The model under review builds one solid part; all positions refer to its coordinate system, in mm. Coordinates: 2 decimals unless noted, no trailing zeros. Loops run counter-clockwise (first coordinate to the right, second up) from the corner with the lowest first, then second, coordinate; pieces in that order, holes last. Notation, with made-up numbers: M -22,-11.75 L 11,-11.75 A33 ccw 11,23.25 Z; hole C -18.5,-37.75 d4. An arc over 180 degrees is marked long. Use one line per item in the form item = value.
```python
from build123d import *

# Parameters (mm, degrees)
F1_W      = 22
F1_H      = 9
F2_DEPTH  = 25
F2_FACE_W = 22
F2_FACE_H = 9
F3_DEPTH  = 100
F4_R      = 5
F5_DEPTH  = 5


with BuildPart() as f2:
    # F1 (on face) → F2 (new body)
    with BuildSketch(Plane.XY):
        Rectangle(F1_W, F1_H)
    extrude(amount=F2_DEPTH)

    # F2_face (on face) → F3 (join)
    with BuildSketch(Plane.XY.offset(25)):
        Rectangle(F2_FACE_W, F2_FACE_H)
    extrude(amount=F3_DEPTH)

    # F4 (on face) → F5 (join)
    with BuildSketch(Plane.XZ.offset(4.5)):
        with Locations((0, 111.583002)):
            Circle(F4_R)
    extrude(amount=F5_DEPTH)


solid = f2.part
```
1. Add section D-D (y = -7.5). State the section outline as (x, z) points, then the cut area to 3 significant figures.
Response values:
outline = C 0,111.58 d10
area = 78.5 mm^2
2. Insertion check: P1, Ø3, axis at x = -2, z = 84.5, coming from the -Y side; P2, Ø1.5, axis at x = -1.5, y = -7.5, coming from the -Z side. Each pin has a flat end and moves straight along its axis. Give the tip position at first contact, or say it passes through.
Response values:
P1 = -4.5
P2 = 106.64
3. Add section A-A (x = 0). State the section outline as (y, z) points.
Response values:
outline = M -9.5,106.58 L -4.5,106.58 L -4.5,0 L 4.5,0 L 4.5,125 L -4.5,125 L -4.5,116.58 L -9.5,116.58 Z
4. The part is to be moulded in two halves that separate along Z. For faces 1 (the face through (-11, 0, 62)), 2 (the face through (0, 0, 125)), 3 (the face through (2.69, -6.96, 115.8)), say which applies: pulls with the +Z half, pulls with the -Z half, needs draft (parallel to the pull), parting line crosses it, or undercut.
Response values:
face_1 = needs draft
face_2 = pulls with the +Z half
face_3 = parting line crosses it
5. Add section B-B (z = 75.5). State the section outline as (x, y) points, then the cut area to 3 significant figures.
Response values:
outline = M -11,-4.5 L 11,-4.5 L 11,4.5 L -11,4.5 Z
area = 198 mm^2
6. Wall thickness on line 1 along Y through (x, z) = (-2.5, 8); line 2 along Z through (x, y) = (-1, -7): over which ranges is each line inside the solid? List them lowest first. Write a range as from..to.
Response values:
line_1 = -4.5..4.5
line_2 = 106.68..116.48
7. Add section C-C (x = 7.5). State the section outline as (y, z) points, then the cut area to 4 significant figures.
Response values:
outline = M -4.5,0 L 4.5,0 L 4.5,125 L -4.5,125 Z
area = 1,125 mm^2
